The listing builds one solid part. Answer for the finished solid, in the listing's coordinates (mm). A direction names the side the tool comes from. Give positions to 0.01 mm unless a question says otherwise; leave off trailing zeros. Order: outer loops, then holes, each group sorted by start corner. A loop starts at its lowest first (then second) coordinate and runs counter-clockwise, first axis right, second up. Notation, with made-up numbers: (47.5, 2.25) - (84.5, 2.25) arc R8 cw to (84.5, 14.25) - close; hole circle Ø5 at (6, 3). An arc over 180 degrees is marked (long way). Write each question's results on one line, items separated by ' | '. Start each with the question number.
1. Flat-ended cylindrical pins translate along their axes: pin 1 (3 mm diameter, centred on x = 93, z = -3.5, fed in from -Y) (3 decimals); pin 2 (3 mm diameter, centred on y = -70, z = 6, fed in from -X) (3 decimals); pin 3 (20.5 mm diameter, centred on x = 133.66, y = -91.6, fed in from -Z). Find the tip coordinate at first contact, or state that the pin passes through.
2. Which of the six approach directions +Z, -Z, +X, -X, +Y, -Y give full straight-line access (tool end or side, diameter ignored) to faces 1 (the face through (63, 0, 8)), 2 (the face through (74.427, -11.143, 9.271)), 3 (the face through (-74.434, -11.131, -9.285))?
3. Section A-A (z = -6) is taken. Give the vertices of the cut face in (x, y), and give its area (3 significant figures).
4. Determine the mould class of faces 4 (the face through (-101.563, -16.995, 9.493)), 5 (the face through (-97.93, -44.92, -1.62)), 6 (the face through (-86.532, -28.96, -9.507)), 7 (the face through (-61.3, 1.3, 6)) for opening direction Y: released by +Y, released by -Y, zero draft, split by the parting line, or undercut.
5. Section B-B (x = 12) is taken. Give the vertices of the cut face in (y, z), and give its area (3 significant figures).
6. Section D-D (x = 108) is taken. Give the vertices of the cut face in (y, z).
7. Section C-C (y = -53) is taken. State how many separate pieces and enclosed holes the cut face has, and give its area (3 significant figures).
8. Find the intervals of material crossed by L1, parallel to X at y = 0, z = -2; L2, parallel to Y at x = 0, z = -1.5; L3, parallel to Y at x = 27.5, z = 7, in increasing order.
from build123d import *

# Parameters (mm, degrees)
SKETCH1_R               = 1.6
BOSS_EXTRUDE1_DEPTH     = 10
SKETCH2_R               = 11.25
SKETCH2_R_2             = 12.75
CUT_EXTRUDE1_DEPTH      = 177.242290049
CUT_EXTRUDE1_DEPTH_BACK = 177.242290049
BOSS_EXTRUDE2_START     = -10
SKETCH2_3_R             = 13.25
SKETCH2_3_R_2           = 11.25
BOSS_EXTRUDE2_DEPTH     = 20
BOSS_EXTRUDE3_START     = 10
SKETCH2_4_R             = 11.25
SKETCH2_4_R_2           = 7.5
BOSS_EXTRUDE3_DEPTH     = 3
BOSS_EXTRUDE4_START     = -10
SKETCH2_5_R             = 14.75
SKETCH2_5_R_2           = 12.75
BOSS_EXTRUDE4_DEPTH     = 20
BOSS_EXTRUDE5_START     = 10
SKETCH2_6_R             = 12.75
SKETCH2_6_R_2           = 1.6
SKETCH2_6_R_3           = 5.5
BOSS_EXTRUDE5_DEPTH     = 2
FILLET1_R               = 10
CUT_EXTRUDE2_START      = 10
SKETCH3_R               = 3
CUT_EXTRUDE2_DEPTH      = 4
CHAMFER1_SIZE           = 1


with BuildPart() as part:
    # Sketch1 → Boss-Extrude1 (new, symmetric)
    with BuildSketch(Plane.XY):
        with BuildLine():
            Line((-75, -10), (75, -10))
            Line((75, -10), (125, -96.602540378))
            ThreePointArc((125, -96.602540378), (138.660254038, -100.262794416), (142.320508076, -86.602540378))
            Line((142.320508076, -86.602540378), (92.320508076, 0))
            ThreePointArc((92.320508076, 0), (85, 7.320508076), (75, 10))
            Line((75, 10), (-75, 10))
            ThreePointArc((-75, 10), (-85, 7.320508076), (-92.320508076, 0))
            Line((-92.320508076, 0), (-117.320508076, -43.301270189))
            ThreePointArc((-117.320508076, -43.301270189), (-113.660254038, -56.961524227), (-100, -53.301270189))
            Line((-100, -53.301270189), (-75, -10))
        make_face()
        Circle(SKETCH1_R, mode=Mode.SUBTRACT)
        with Locations((-60, 0)):
            Circle(SKETCH1_R, mode=Mode.SUBTRACT)
        with Locations((-30, 0)):
            Circle(SKETCH1_R, mode=Mode.SUBTRACT)
        with Locations((30, 0)):
            Circle(SKETCH1_R, mode=Mode.SUBTRACT)
        with Locations((60, 0)):
            Circle(SKETCH1_R, mode=Mode.SUBTRACT)
    extrude(amount=BOSS_EXTRUDE1_DEPTH, both=True)

    # Sketch2 → Cut-Extrude1 (cut, two sides)
    with BuildSketch(Plane.XY) as cut_extrude1_sk:
        with Locations((-108.660254038, -48.301270189)):
            Circle(SKETCH2_R)
        with Locations((133.660254038, -91.602540378)):
            Circle(SKETCH2_R_2)
    extrude(amount=CUT_EXTRUDE1_DEPTH, mode=Mode.SUBTRACT)
    extrude(cut_extrude1_sk.sketch, amount=-CUT_EXTRUDE1_DEPTH_BACK, mode=Mode.SUBTRACT)

    # Sketch2<3> → Boss-Extrude2 (add)
    with BuildSketch(Plane.XY.offset(BOSS_EXTRUDE2_START)):
        with Locations((-108.660254038, -48.301270189)):
            Circle(SKETCH2_3_R)
        with Locations((-108.660254038, -48.301270189)):
            Circle(SKETCH2_3_R_2, mode=Mode.SUBTRACT)
    extrude(amount=BOSS_EXTRUDE2_DEPTH)

    # Sketch2<4> → Boss-Extrude3 (add)
    with BuildSketch(Plane.XY.offset(BOSS_EXTRUDE3_START)):
        with Locations((-108.660254038, -48.301270189)):
            Circle(SKETCH2_4_R)
        with Locations(Location((-108.660254038, -48.301270189, 0), (0, 0, 180))):
            Circle(SKETCH2_4_R_2, mode=Mode.SUBTRACT)
    extrude(amount=-BOSS_EXTRUDE3_DEPTH)

    # Sketch2<5> → Boss-Extrude4 (add)
    with BuildSketch(Plane.XY.offset(BOSS_EXTRUDE4_START)):
        with Locations((133.660254038, -91.602540378)):
            Circle(SKETCH2_5_R)
        with Locations((133.660254038, -91.602540378)):
            Circle(SKETCH2_5_R_2, mode=Mode.SUBTRACT)
    extrude(amount=BOSS_EXTRUDE4_DEPTH)

    # Sketch2<6> → Boss-Extrude5 (add)
    with BuildSketch(Plane.XY.offset(BOSS_EXTRUDE5_START)):
        with Locations((133.660254038, -91.602540378)):
            Circle(SKETCH2_6_R)
        with Locations(Location((125.160254038, -91.602540378, 0), (0, 0, 180))):
            Circle(SKETCH2_6_R_2, mode=Mode.SUBTRACT)
        with Locations(Location((133.660254038, -91.602540378, 0), (0, 0, 180))):
            Circle(SKETCH2_6_R_3, mode=Mode.SUBTRACT)
        with Locations(Location((142.160254038, -91.602540378, 0), (0, 0, 180))):
            Circle(SKETCH2_6_R_2, mode=Mode.SUBTRACT)
    extrude(amount=-BOSS_EXTRUDE5_DEPTH)

    # Fillet1
    fillet1_edges = [part.edges().sort_by_distance(p)[0] for p in [
        (136.899195965, -77.212552359, 0),
        (119.578687889, -87.212552359, 0),
        (75, -10, 0),
        (-75, -10, 0),
        (-112.974173413, -35.773197727, 0),
        (-95.653665337, -45.773197727, 0),
    ]]
    fillet(fillet1_edges, radius=FILLET1_R)

    # Sketch3 → Cut-Extrude2 (cut)
    with BuildSketch(Plane.XY.offset(CUT_EXTRUDE2_START)):
        with Locations(Location((-60, 0, 0), (0, 0, 180))):
            Circle(SKETCH3_R)
        with Locations(Location((-30, 0, 0), (0, 0, 180))):
            Circle(SKETCH3_R)
        with Locations(Location((0, 0, 0), (0, 0, 180))):
            Circle(SKETCH3_R)
        with Locations(Location((30, 0, 0), (0, 0, 180))):
            Circle(SKETCH3_R)
        with Locations(Location((60, 0, 0), (0, 0, 180))):
            Circle(SKETCH3_R)
    extrude(amount=-CUT_EXTRUDE2_DEPTH, mode=Mode.SUBTRACT)

    # Chamfer1
    chamfer1_edges = [part.edges().sort_by_distance(p)[0] for p in [
        (-101.85653165, -16.516877333, -10),
        (-85, 7.320508076, -10),
        (0, 10, -10),
        (85, 7.320508076, -10),
        (141.035254038, -104.376415084, 10),
        (141.035254038, -104.376415084, -10),
        (113.675627248, -36.988151408, -10),
        (113.675627248, -36.988151408, 10),
        (-115.285254038, -59.776106789, -10),
        (-115.285254038, -59.776106789, 10),
        (-85.979399248, -29.016877333, -10),
        (-85.979399248, -29.016877333, 10),
        (97.798494845, -49.488151408, 10),
        (97.798494845, -49.488151408, -10),
        (0, -10, -10),
        (0, -10, 10),
        (137.005608205, -76.413071632, 10),
        (137.005608205, -76.413071632, -10),
        (-113.022539154, -35.145386139, -10),
        (-113.022539154, -35.145386139, 10),
        (-95.085781683, -45.501177894, 10),
        (-95.085781683, -45.501177894, -10),
        (118.83311115, -86.904967699, -10),
        (118.83311115, -86.904967699, 10),
        (74.226497308, -11.339745962, -10),
        (74.226497308, -11.339745962, 10),
        (-74.226497308, -11.339745962, -10),
        (-74.226497308, -11.339745962, 10),
        (85, 7.320508076, 10),
        (0, 10, 10),
        (-85, 7.320508076, 10),
        (-101.85653165, -16.516877333, 10),
    ]]
    chamfer(chamfer1_edges, length=CHAMFER1_SIZE)


solid = part.part
Reported:
1) pin 1: y = -43.775 | pin 2: x = 108.775 | pin 3: z = 8
2) face 1: +Z | face 2: +Z, -Y | face 3: -Z, -Y
3) outline: (-115.15, -36.75) arc R13.25 ccw (long way) to (-95.41, -48.15) arc R10 cw to (-94.07, -43.03) - (-77.89, -15) arc R10 cw to (-69.23, -10) - (69.23, -10) arc R10 cw to (77.89, -15) - (117.71, -83.98) arc R10 cw to (118.99, -90.04) arc R14.75 ccw (long way) to (139.64, -78.12) arc R10 cw to (135.03, -73.98) - (92.32, 0) arc R20 ccw to (75, 10) - (-75, 10) arc R20 ccw to (-92.32, 0) - (-111.39, -33.03) arc R10 cw to start; hole circle Ø22.5 at (-108.66, -48.3); hole circle Ø3.2 at (-60, 0); hole circle Ø3.2 at (-30, 0); hole circle Ø3.2 at (0, 0); hole circle Ø3.2 at (30, 0); hole circle Ø3.2 at (60, 0); hole circle Ø25.5 at (133.66, -91.6) | area: 6,210 mm²
4) face 4: released by +Y | face 5: undercut | face 6: released by -Y | face 7: undercut
5) outline: (-10, -9) - (-9, -10) - (9, -10) - (10, -9) - (10, 9) - (9, 10) - (-9, 10) - (-10, 9) - close | area: 398 mm²
6) outline: (-67.16, -9) - (-65.16, -10) - (-29.16, -10) - (-27.16, -9) - (-27.16, 9) - (-29.16, 10) - (-65.16, 10) - (-67.16, 9) - close
7) separate pieces: 3 | enclosed holes: 0 | area: 570 mm²
8) L1: -92.32 to -61.6, -58.4 to -31.6, -28.4 to -1.6, 1.6 to 28.4, 31.6 to 58.4, 61.6 to 92.32 | L2: -10 to -1.6, 1.6 to 10 | L3: -10 to -1.66, 1.66 to 10
